Autodesk Inventor part; units mm, degrees
ref_plane "YZ Plane" through (0, 0, 0) normal (1, 0, 0) x (0, 1, 0)
ref_plane "XZ Plane" through (0, 0, 0) normal (0, 1, 0) x (-1, 0, 0)
ref_plane "XY Plane" through (0, 0, 0) normal (0, 0, 1) x (1, 0, 0)
sketch "Sketch1" plane through (0, 0, 0) normal (0, 0, 1) x (1, 0, 0)
  line L0 (0, 0) -> (0, -25.4)
  line L1 (0, -25.4) -> (50.8, -25.4)
  line L2 (50.8, -25.4) -> (50.8, 0)
  line L3 (50.8, 0) -> (0, 0)
  dimension "d0" = 25.4
  dimension "d1" = 50.8
extrude "Extrusion1" add sketch "Sketch1" along normal blind 342.9
sketch "Sketch3" plane through (50.8, -25.4, 0) normal (1, 0, 0) x (0, 0, -1)
  line L0 (0, 0) -> (-342.9, 0)
  line L1 (-171.45, 0) -> (-196.8396, 0)
  line L2 (-196.8396, 0) -> (-146.0396, 0)
  arc A0 (-146.0396, 0) -> (-196.8396, 0) centre (-171.4396, -41.9008) ccw
  line L3 (-171.45, 0) -> (-171.45, 25.4)
  point P0 (0, 25.4)
  dimension "d10" = 50.8
extrude "Extrusion2" cut sketch "Sketch3" against normal through all
properties part number "connectingthing" material "Aluminum 6061"
Geometry check sheet. Reference: the model listing, model coordinates, mm. Coordinates: 2 decimals unless noted, no trailing zeros. Order: outer loops, then holes, each group sorted by start corner. A loop starts at its lowest first (then second) coordinate and runs counter-clockwise, first axis right, second up. Notation, with made-up numbers: (11.5, 9) - (30.5, 9) arc R27 cw to (30.5, 42) - close; hole circle Ø11 at (13, 7). An arc over 180 degrees is marked (long way). Answer in a Markdown table with one row per item. Add a question column.
1) Gauge pin test, flat end, axial feed: P1, Ø2, axis at x = 31.5, z = 203.5, coming from the +Y side. Record the tip position at first contact, or that the pin passes through.
2) Cross-section at B-B, the plane x = 32. Record the cut outline in (y, z).
3) Cross-section at C-C, the plane z = 166. Record the cut outline in (x, y).
4) Material ranges on line 1 along Z through (x, y) = (40, -24.25); line 2 along Z through (x, y) = (9, -22); line 3 along Y through (x, z) = (42, 147), recorded low to high. Write a range as [from, to].
5) Release check for a two-part mould opening along Z. For faces 1 (the cylindrical face through (25.756, -18.304, 171.066)), 2 (the flat face through (26, 0, 169)), 3 (the flat face through (25, -13, 0)) record: +Z half, -Z half, draft (parallel to the pull), parting line (faces both ways), or undercut.
6) Cross-section at A-A, the plane y = -21.5. Record the cut outline in (x, z), then the cut area to 3 significant figures.
Check result:
| question | item | result |
|---|---|---|
| 1 | P1 | stops at y = 0 |
| 2 | outline | (-25.4, 0) - (0, 0) - (0, 342.9) - (-25.4, 342.9) - (-25.4, 196.84) arc R49 cw to (-25.4, 146.04) - close |
| 3 | outline | (0, -18.61) - (50.8, -18.61) - (50.8, 0) - (0, 0) - close |
| 4 | line 1 | z = [0, 148.04], [194.84, 342.9] |
| 4 | line 2 | z = [0, 152.77], [190.11, 342.9] |
| 4 | line 3 | y = [-24.83, 0] |
| 5 | face 1 | undercut |
| 5 | face 2 | draft |
| 5 | face 3 | -Z half |
| 6 | outline | (0, 0) - (50.8, 0) - (50.8, 154.03) - (0, 154.03) - close; (0, 188.85) - (50.8, 188.85) - (50.8, 342.9) - (0, 342.9) - close |
| 6 | area | 15,700 mm² |
